Check sheet for the drawn part. Datum: minimum x, y, z corner. Units: mm. A direction names the side the tool comes from. Give positions to 0.01 mm unless a question says otherwise; leave off trailing zeros. Loops run counter-clockwise (first coordinate to the right, second up) from the corner with the lowest first, then second, coordinate; pieces in that order, holes last.
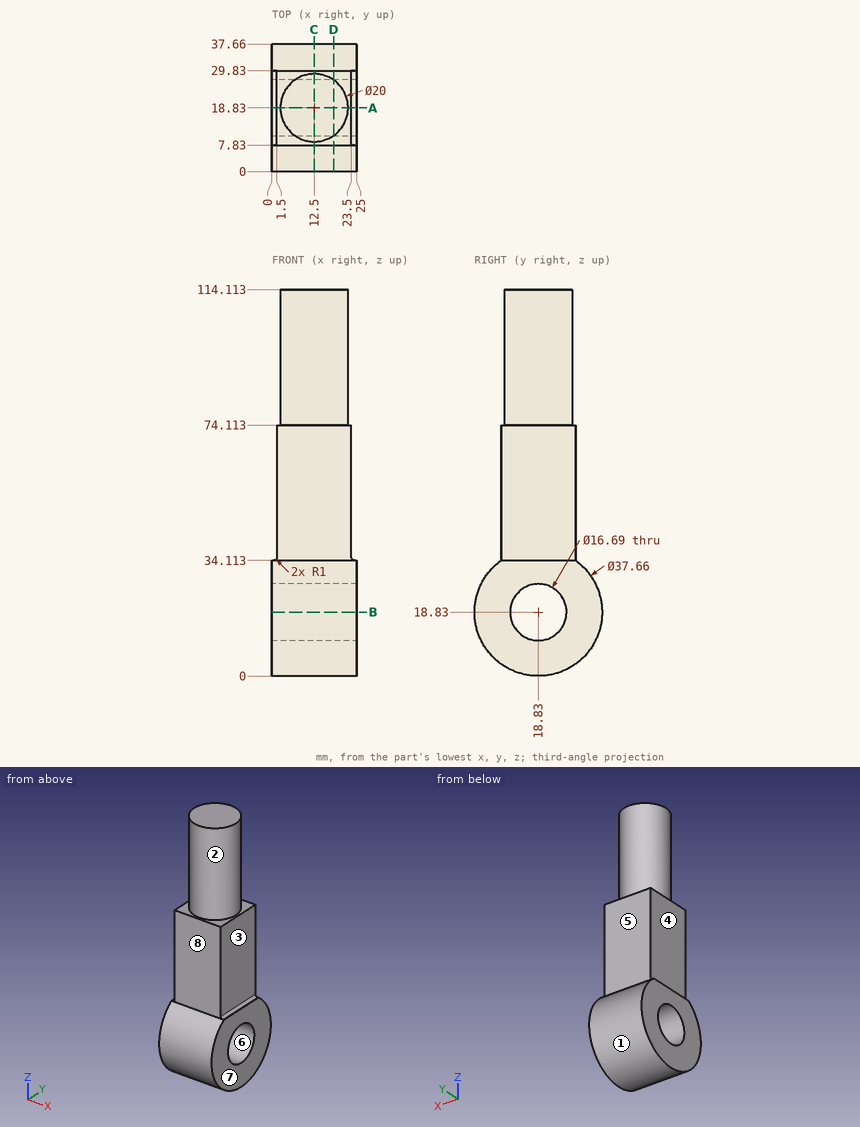
1) Depth check by flat-ended pin: P1, Ø10, axis at y = 18.83, z = 18.83, coming from the +X side; P2, Ø4, axis at x = 7, z = 35, coming from the +Y side; P3, Ø2, axis at x = 9.5, y = 30.5, coming from the +Z side; P4, Ø3, axis at x = 14, z = 69.5, coming from the +Y side. Enter the tip coordinate at first touch or a pass-through.
2) Scan lines: line 1 along Y through (x, z) = (10, 18.83) (3 decimals); line 2 along Y through (x, z) = (10.5, 13); line 3 along X through (y, z) = (12.5, 71). Record each from-to range of solid material in increasing order.
3) Sectioned sample at A-A on y = 18.83. Enter the section's corners in (x, z) (3 decimals).
4) Tool access check on the marked faces 1, 2, 3 and 4. Record the directions out of +Z, -Z, +X, -X, +Y, -Y that give a thin tool (end or side, any length) a straight path to the whole face; none if there is none.
5) Mould release check, pull along Y, two halves, no side actions. Record for the marked faces 5, 6, 7 and 8: +Y half, -Y half, draft (parallel to the pull), parting line (faces both ways), or undercut.
6) Sectioned sample at B-B on z = 18.83. Enter the section's corners in (x, y) (3 decimals).
7) Sectioned sample at D-D on x = 18.25. Enter the section's corners in (y, z) (1 decimal), plus the area to 3 significant figures.
8) Sectioned sample at C-C on x = 12.5. Enter the section's corners in (y, z) (3 decimals), plus the area to 3 significant figures.
Determined:
1. P1: passes through
1. P2: stops at y = 31.23
1. P3: stops at z = 74.11
1. P4: stops at y = 29.83
2. line 1: y = 0 to 10.485, 27.175 to 37.66
2. line 2: y = 0.93 to 12.86, 24.8 to 36.73
2. line 3: x = 1.5 to 23.5
3. outline: (0, 0) - (25, 0) - (25, 10.485) - (0, 10.485) - close; (0, 27.175) - (25, 27.175) - (25, 34.113) - (24.5, 34.113) arc R1 cw to (23.5, 35.113) - (23.5, 74.113) - (22.5, 74.113) - (22.5, 114.113) - (2.5, 114.113) - (2.5, 74.113) - (1.5, 74.113) - (1.5, 35.113) arc R1 cw to (0.5, 34.113) - (0, 34.113) - close
4. face 1: +X, -X
4. face 2: +Z
4. face 3: +Z, +X, +Y, -Y
4. face 4: +Z, -X, +Y, -Y
5. face 5: +Y half
5. face 6: undercut
5. face 7: draft
5. face 8: -Y half
6. outline: (0, 0) - (25, 0) - (25, 10.485) - (0, 10.485) - close; (0, 27.175) - (25, 27.175) - (25, 37.66) - (0, 37.66) - close
7. outline: (7.8, 34.1) arc R18.8 ccw (long way) to (29.8, 34.1) - (29.8, 74.1) - (27, 74.1) - (27, 114.1) - (10.6, 114.1) - (10.6, 74.1) - (7.8, 74.1) - close; hole circle Ø16.7 at (18.8, 18.8)
7. area: 2,380 mm2
8. outline: (7.83, 34.113) arc R18.83 ccw (long way) to (29.83, 34.113) - (29.83, 74.113) - (28.83, 74.113) - (28.83, 114.113) - (8.83, 114.113) - (8.83, 74.113) - (7.83, 74.113) - close; hole circle Ø16.69 at (18.83, 18.83)
8. area: 2,520 mm2
